Answer from the drawing. Dimensions are ordinates in mm from the lowest x, y and z of the part. A direction names the side the tool comes from. Give positions to 0.01 mm unless a question says otherwise; leave off trailing zeros. Loops run counter-clockwise (first coordinate to the right, second up) from the corner with the lowest first, then second, coordinate; pieces in that order, holes last. Notation, with made-up numbers: (-1.75, 55.5) - (47.25, 55.5) arc R31 ccw to (47.25, 93.5) - close; hole circle Ø6 at (41, -14). An arc over 180 degrees is marked (long way). Answer as CSV lines item,"result". Start each with the question number.
1) A cutting plane is placed at B-B (z = 16). Determine the outline of the cut face in (x, y), and give its area (3 significant figures).
2) Find the intervals of material crossed by line 1 along Z through (x, y) = (7, 9); line 2 along X through (y, z) = (33, 46.5); line 3 along Y through (x, z) = (10, 46), in increasing order.
3) A cutting plane is placed at C-C (y = 12.5). Determine the outline of the cut face in (x, z), and give its area (3 significant figures).
4) A cutting plane is placed at A-A (x = 5.5). Determine the outline of the cut face in (y, z).
5) Flat-ended cylindrical pins translate along their axes: pin 1 (5 mm diameter, centred on x = 13.5, z = 13.5, fed in from +Y); pin 2 (5 mm diameter, centred on y = 8.5, z = 36.5, fed in from -X); pin 3 (20 mm diameter, centred on y = 40, z = 26.5, fed in from -X). Find the tip coordinate at first contact, or state that the pin passes through.
6) For the marked faces 5, 6, 7, 8 and 9, determine the directions among +Z, -Z, +X, -X, +Y, -Y from which every point of the face is accessible in a straight line to the end or side of a thin tool.
7) For a pull along Z with two mould halves and no side action, classify the marked faces 1, 2, 3 and 4 as pulls with the +Z half, pulls with the -Z half, needs draft (parallel to the pull), parting line crosses it, or undercut.
8) A cutting plane is placed at D-D (z = 41). Determine the outline of the cut face in (x, y).
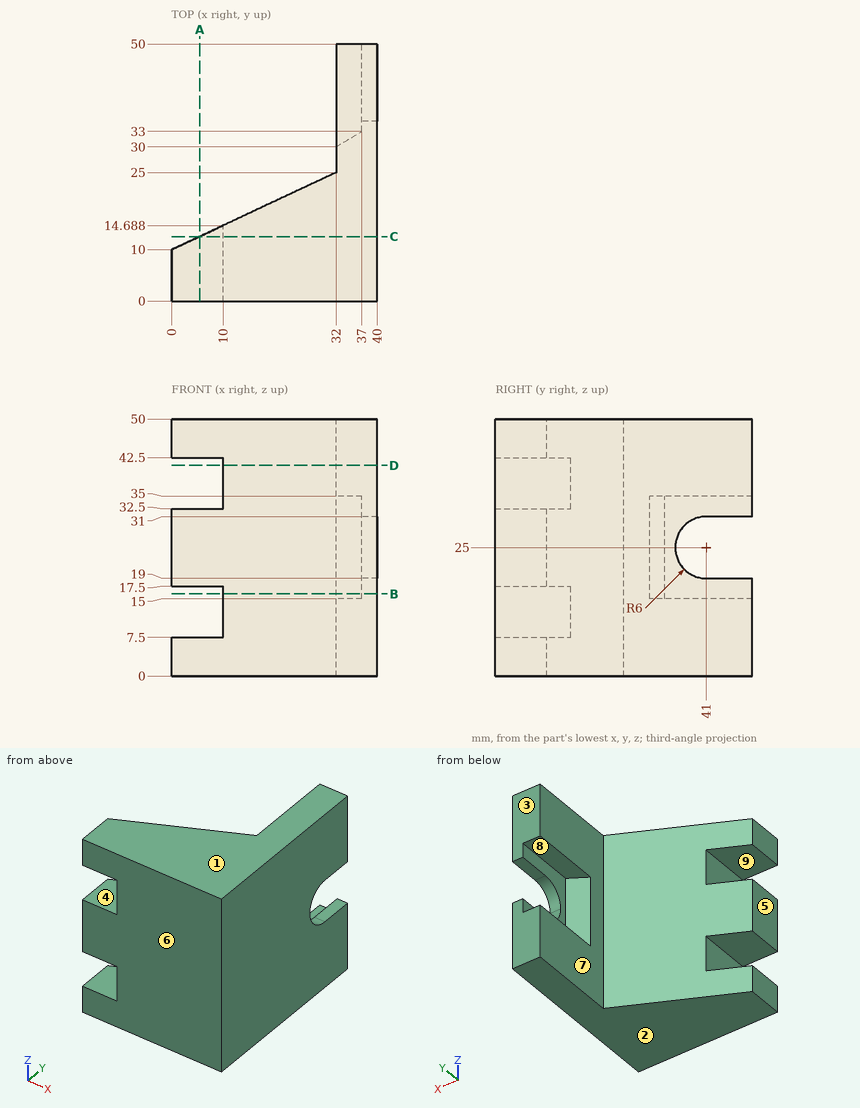
Ans:
1,outline,"(10, 0) - (40, 0) - (40, 50) - (37, 50) - (37, 33) - (32, 30) - (32, 25) - (10, 14.69) - close"
1,area,"744 mm2"
2,line 1,"0 to 7.5, 17.5 to 32.5, 42.5 to 50"
2,line 2,"32 to 40"
2,line 3,"0 to 14.69"
3,outline,"(5.33, 0) - (40, 0) - (40, 50) - (5.33, 50) - (5.33, 42.5) - (10, 42.5) - (10, 32.5) - (5.33, 32.5) - (5.33, 17.5) - (10, 17.5) - (10, 7.5) - (5.33, 7.5) - close"
3,area,"1,640 mm2"
4,outline,"(0, 0) - (12.58, 0) - (12.58, 7.5) - (0, 7.5) - close; (0, 17.5) - (12.58, 17.5) - (12.58, 32.5) - (0, 32.5) - close; (0, 42.5) - (12.58, 42.5) - (12.58, 50) - (0, 50) - close"
5,pin 1,"y = 17.5"
5,pin 2,"x = 10"
5,pin 3,"x = 32"
6,face 5,"+Z, -Z, -X, +Y, -Y"
6,face 6,"+Z, -Z, +X, -X, -Y"
6,face 7,"+Z, -Z, -X, +Y"
6,face 8,"-X, +Y"
6,face 9,"-X, +Y, -Y"
7,face 1,"pulls with the +Z half"
7,face 2,"pulls with the -Z half"
7,face 3,"needs draft"
7,face 4,"undercut"
8,outline,"(10, 0) - (40, 0) - (40, 50) - (32, 50) - (32, 25) - (10, 14.69) - close"
